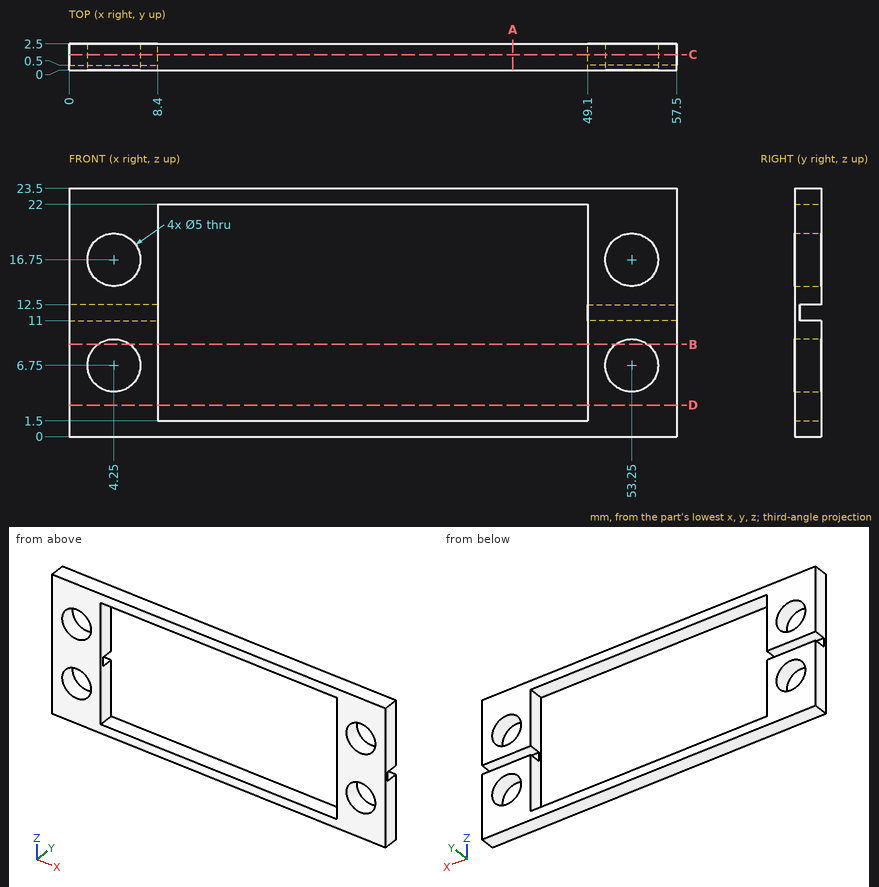
Check sheet for the drawn part. Datum: minimum x, y, z corner. Units: mm. Round coordinates to 2 decimals unless told otherwise and drop trailing zeros. Loops run counter-clockwise (first coordinate to the right, second up) from the corner with the lowest first, then second, coordinate; pieces in that order, holes last. Notation, with made-up numbers: (23.25, 42.5) -> (65.25, 42.5) arc R24 ccw to (65.25, 59.5) -> close; hole circle Ø11 at (84.25, 79). An arc over 180 degrees is marked (long way). Put each result on its own line as item: value. Start each with the question number.
1. Section check B-B (z = 8.75). Enter the section's corners in (x, y).
2. Gauge pin test, flat ends, axial feed: pin 1 (0.8 mm diameter, centred on y = 0.5, z = 10.5, fed in from -X); pin 2 (4 mm diameter, centred on x = 4.25, z = 6.75, fed in from -Y). Record the tip position at first contact, or that the pin passes through.
3. Section check C-C (y = 1.5). Enter the section's corners in (x, z), plus the area to 3 significant figures.
4. Scan lines: probe 1 along X at (y, z) = (0.55, 6.75); probe 2 along Z at (x, y) = (4.25, 1.15); probe 3 along Z at (x, y) = (34.5, 1.75). Record each from-to range of solid material in increasing order.
5. Section check A-A (x = 42). Enter the section's corners in (y, z).
6. Section check D-D (z = 3). Enter the section's corners in (x, y).
Findings:
1. outline: (0, 0) -> (2.75, 0) -> (2.75, 2.5) -> (0, 2.5) -> close; (5.75, 0) -> (8.4, 0) -> (8.4, 2.5) -> (5.75, 2.5) -> close; (49.1, 0) -> (51.75, 0) -> (51.75, 2.5) -> (49.1, 2.5) -> close; (54.75, 0) -> (57.5, 0) -> (57.5, 2.5) -> (54.75, 2.5) -> close
2. pin 1: stops at x = 0
2. pin 2: passes through
3. outline: (0, 0) -> (57.5, 0) -> (57.5, 11) -> (49.1, 11) -> (49.1, 1.5) -> (8.4, 1.5) -> (8.4, 11) -> (0, 11) -> close; (0, 12.5) -> (8.4, 12.5) -> (8.4, 22) -> (49.1, 22) -> (49.1, 12.5) -> (57.5, 12.5) -> (57.5, 23.5) -> (0, 23.5) -> close; hole circle Ø5 at (4.25, 6.75); hole circle Ø5 at (4.25, 16.75); hole circle Ø5 at (53.25, 6.75); hole circle Ø5 at (53.25, 16.75)
3. area: 413 mm^2
4. probe 1: x = 0 to 1.75, 6.75 to 8.4, 49.1 to 50.75, 55.75 to 57.5
4. probe 2: z = 0 to 4.25, 9.25 to 11, 12.5 to 14.25, 19.25 to 23.5
4. probe 3: z = 0 to 1.5, 22 to 23.5
5. outline: (0, 0) -> (2.5, 0) -> (2.5, 1.5) -> (0, 1.5) -> close; (0, 22) -> (2.5, 22) -> (2.5, 23.5) -> (0, 23.5) -> close
6. outline: (0, 0) -> (8.4, 0) -> (8.4, 2.5) -> (0, 2.5) -> close; (49.1, 0) -> (57.5, 0) -> (57.5, 2.5) -> (49.1, 2.5) -> close
